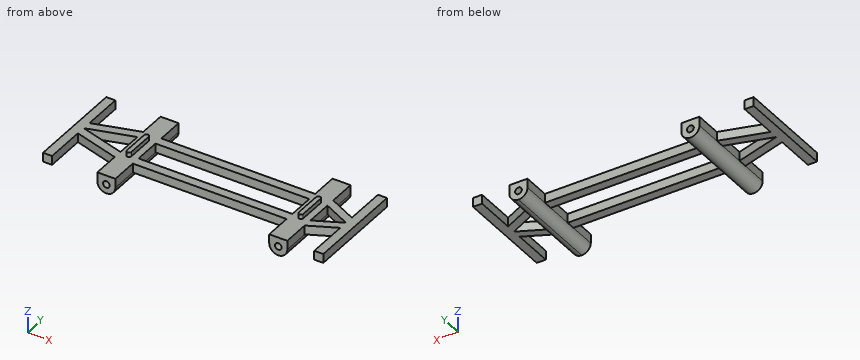
from build123d import *

# Parameters (mm, degrees)
F1_DEPTH  = 2
F3_DEPTH  = 1
F5_DEPTH  = 21.8461783077
F6_W      = 4
F6_H      = 21.8461783077
F7_DEPTH  = 2
F8_R      = 1.99999
F10_R     = 0.75
F9_R      = 0.75
F11_DEPTH = 21.9240891538


# Not quite as in the source:
# - a fillet or chamfer is up to 0.001 mm smaller than in the source, because OpenCascade refuses the exact size


with BuildPart() as f1:
    # F0 (on Top) → F1 (new body)
    with BuildSketch(Plane.XY):
        Polygon((0, -11), (0, 0), (0, 11), (-2, 11), (-2, 2), (-8, 4.9230891538), (-8, 10.9230891538), (-12, 10.9230891538), (-12, 4.9230891538), (-29, 4.9230891538), (-46, 4.9230891538), (-46, 10.9230891538), (-50, 10.9230891538), (-50, 4.9230891538), (-60, 2), (-60, 10.9230891538), (-62, 10.9230891538), (-62, -10.9230891538), (-60, -10.9230891538), (-60, -2), (-50, -4.9230891538), (-50, -10.9230891538), (-46, -10.9230891538), (-46, -4.9230891538), (-29, -4.9230891538), (-12, -4.9230891538), (-12, -10.9230891538), (-8, -10.9230891538), (-8, -4.9230891538), (-2, -2), (-2, -11), align=None)
        Polygon((-60, 0), (-50, 2.9230891538), (-50, -2.9230891538), align=None, mode=Mode.SUBTRACT)
        Polygon((-12, 2.9230891538), (-12, 0), (-12, -2.9230891538), (-29, -2.9230891538), (-46, -2.9230891538), (-46, 0), (-46, 2.9230891538), (-29, 2.9230891538), align=None, mode=Mode.SUBTRACT)
        Polygon((-8, 2.9230891538), (-2, 0), (-8, -2.9230891538), (-8, 0), align=None, mode=Mode.SUBTRACT)
    extrude(amount=F1_DEPTH)

    # F2 (on face) → F3 (join)
    with BuildSketch(Plane.XY.offset(2)):
        with BuildLine():
            Line((-47.5, -3.0769108462), (-47.5, 2.9230891538))
            ThreePointArc((-47.5, 2.9230891538), (-48, 3.4230891538), (-48.5, 2.9230891538))
            Line((-48.5, 2.9230891538), (-48.5, -3.0769108462))
            ThreePointArc((-48.5, -3.0769108462), (-48, -3.5769108462), (-47.5, -3.0769108462))
        make_face()
        with BuildLine():
            Line((-9.5, -3.0769108462), (-9.5, 2.9230891538))
            ThreePointArc((-9.5, 2.9230891538), (-10, 3.4230891538), (-10.5, 2.9230891538))
            Line((-10.5, 2.9230891538), (-10.5, -3.0769108462))
            ThreePointArc((-10.5, -3.0769108462), (-10, -3.5769108462), (-9.5, -3.0769108462))
        make_face()
    extrude(amount=F3_DEPTH)

    # F4 (on face) → F5 (join, through all)
    with BuildSketch(Plane.XZ.offset(10.9230891538)):
        with BuildLine():
            Line((-46, 0), (-50, 0))
            ThreePointArc((-50, 0), (-48, -2), (-46, 0))
        make_face()
    extrude(amount=-F5_DEPTH)

    # F6 (on face) → F7 (join)
    with BuildSketch(Plane(origin=(0, 0, 0), x_dir=(1, 0, 0), z_dir=(0, 0, -1))):
        with Locations((-10, 0)):
            Rectangle(F6_W, F6_H)
    extrude(amount=F7_DEPTH)

    # F8 (radius 2 in the source; OpenCascade refuses exactly that, so slightly less here)
    f8_edges = [f1.edges().sort_by_distance(p)[0] for p in [
        (-12, 0, -2),
        (-8, 0, -2),
    ]]
    fillet(f8_edges, radius=F8_R)

    # F10 (on face) + F9 (on face) → F11 (cut, through all)
    with BuildSketch(Plane.XZ.offset(10.9230891538)):
        with Locations((-10, 0)):
            Circle(F10_R)
    with BuildSketch(Plane.XZ.offset(10.9230891538)):
        with Locations((-48, 0)):
            Circle(F9_R)
    extrude(amount=-F11_DEPTH, mode=Mode.SUBTRACT)


solid = f1.part
The model under review builds one solid part; all positions refer to its coordinate system, in mm. Round coordinates to 2 decimals unless told otherwise and drop trailing zeros. Write each loop counter-clockwise with the first axis right and the second up, starting at its lowest first coordinate (ties: lowest second). Pieces come first, ordered by that corner, then holes. Notation, with made-up numbers: M 42.25,4 L 54.25,4 A25 cw 54.25,18 Z; hole C 62.5,41 d3. An arc over 180 degrees is marked long. Use a Markdown table: item, result. Add a question column.
Q1. We need section A-A, the plane y = -8.25. Count the separate pieces of the cut face and the enclosed holes in it, plus the area to 3 significant figures.
Q2. Insertion check: pin 1 (1 mm diameter, centred on x = -23, z = 1, fed in from +Y); pin 2 (2.5 mm diameter, centred on x = -4.5, y = 0, fed in from -Z); pin 3 (1 mm diameter, centred on x = -30, z = 1.5, fed in from -Y); pin 4 (5 mm diameter, centred on x = -46, y = 1, fed in from -Z). Each pin has a flat end and moves straight along its axis. Give the tip position at first contact, or say it passes through.
Q3. To check wall thickness, follow line 1 (Z direction, x = -48, y = -2.5); line 2 (Z direction, x = -48, y = -5); line 3 (X direction, y = -5, z = -0.65). State the ranges of each line that lie inside material, in increasing order.
Q4. We need section B-B, the plane x = -7. State the section outline as (y, z) points, plus the area to 3 significant figures.
Findings below:
| question | item | result |
|---|---|---|
| 1 | separate pieces | 4 |
| 1 | enclosed holes | 2 |
| 1 | area | 33.0 mm² |
| 2 | pin 1 | stops at y = 4.92 |
| 2 | pin 2 | stops at z = 0 |
| 2 | pin 3 | stops at y = -4.92 |
| 2 | pin 4 | stops at z = -2 |
| 3 | line 1 | z = -2 to -0.75, 0.75 to 3 |
| 3 | line 2 | z = -2 to -0.75, 0.75 to 2 |
| 3 | line 3 | x = -49.89 to -48.37, -47.63 to -46.11, -11.89 to -10.37, -9.63 to -8.11 |
| 4 | outline | M -4.44,0 L -2.44,0 L -2.44,2 L -4.44,2 Z; M 2.44,0 L 4.44,0 L 4.44,2 L 2.44,2 Z |
| 4 | area | 8.00 mm² |
